Input: part model. Units: mm. Frame: model coordinates. A direction names the side the tool comes from. Coordinates: 2 decimals unless noted, no trailing zeros. Order: outer loops, then holes, each group sorted by start corner. A loop starts at its lowest first (then second) coordinate and runs counter-clockwise, first axis right, second up.
Autodesk Inventor part; units mm, degrees
ref_plane "YZ Plane" through (0, 0, 0) normal (1, 0, 0) x (0, 1, 0)
ref_plane "XZ Plane" through (0, 0, 0) normal (0, 1, 0) x (-1, 0, 0)
ref_plane "XY Plane" through (0, 0, 0) normal (0, 0, 1) x (1, 0, 0)
sketch "Sketch1" plane through (0, 0, 0) normal (0, 0, 1) x (1, 0, 0)
  circle A0 centre (0, 0) radius 50
  dimension "d0" = 100
extrude "Extrusion1" add sketch "Sketch1" along normal mid plane 100
sketch "Sketch2" plane through (0, 0, -50) normal (0, 0, -1) x (-1, 0, 0)
  circle A0 centre (0, 0) radius 45
  dimension "d3" = 90
extrude "Extrusion2" cut sketch "Sketch2" against normal blind 95
sketch "Sketch5" plane through (0, 0, 50) normal (0, 0, 1) x (1, 0, 0)
  point P0 (0, 0)
sketch "Sketch7" plane through (0, 0, 50) normal (0, 0, 1) x (1, 0, 0)
  arc A0 (50, 0) -> (50, 0) centre (0, 0) ccw construction
  circle A1 centre (0, 0) radius 50 construction
sketch "Sketch8" plane through (0, 0, -50) normal (0, 0, -1) x (-1, 0, 0)
  arc A0 (48.2963, -12.941) -> (48.2963, 12.941) centre (0, 0) ccw
  line L0 (0, 0) -> (50, 0) construction
  line L1 (48.2963, 12.941) -> (68.2963, 12.941)
  line L2 (68.2963, 12.941) -> (68.2963, -12.941)
  line L3 (68.2963, -12.941) -> (48.2963, -12.941)
  line L4 (48.2963, 12.941) -> (-48.2963, 12.941) construction
  line L5 (48.2963, -12.941) -> (-48.2963, -12.941) construction
  circle A1 centre (0, 0) radius 50 construction
  arc A2 (-48.2963, 12.941) -> (-48.2963, -12.941) centre (0, 0) ccw
  line L6 (-48.2963, -12.941) -> (-68.2963, -12.941)
  line L7 (-68.2963, -12.941) -> (-68.2963, 12.941)
  line L8 (-68.2963, 12.941) -> (-48.2963, 12.941)
  dimension "d31" = 50
  dimension "d34" = 20
  dimension "d35" = 20
extrude "Extrusion5" add sketch "Sketch8" against normal blind 10
sketch "Sketch9" plane through (0, 0, 50) normal (0, 0, 1) x (1, 0, 0)
  point P0 (0, 0)
sketch "Sketch10" plane through (0, 0, 50) normal (0, 0, 1) x (1, 0, 0)
  line L0 (-68.2963, -12.941) -> (-68.2963, 12.941) construction
  line L1 (-68.2963, -12.941) -> (-48.4721, 12.941) construction
  line L2 (-68.2963, 12.941) -> (-48.4721, -12.941) construction
  line L3 (48.2963, 12.941) -> (68.2963, 12.941) construction
  line L4 (48.2963, -12.941) -> (68.2963, 12.941) construction
  line L5 (68.2963, 12.941) -> (68.2963, -12.941) construction
  arc A0 (48.2963, -12.941) -> (48.2963, 12.941) centre (0, 0) ccw construction
  line L6 (68.2963, -12.941) -> (48.2963, 12.941) construction
  point P0 (-58.3842, 0)
  point P1 (58.2963, 0)
hole "Hole2" at (-58.3842, 0, 50) at (58.2963, 0, 50) direction (0, 0, -1) diameter 8 end through all counterbore diameter 11 counterbore depth 6.5
sketch "Sketch11" plane through (-68.2963, -12.941, -50) normal (0, -1, 0) x (1, 0, 0)
  line L0 (20, 0) -> (116.5926, 0) construction
  line L1 (118.2963, 100) -> (18.2963, 100) construction
  line L2 (20, 0) -> (118.2963, 100) construction
  line L3 (118.2963, 100) -> (18.2963, 100) construction
  line L4 (116.5926, 10) -> (116.5926, 0) construction
  line L5 (18.2963, 100) -> (116.5926, 0) construction
  point P0 (68.2963, 50)
  point P1 (68.2963, 50)
hole "Hole3" at (0, -12.941, 0) direction (0, 1, 0) diameter 8 end through all
sketch "Sketch12" plane through (0, 0, 50) normal (0, 0, 1) x (1, 0, 0)
  circle A0 centre (0, 0) radius 42
  circle A1 centre (0, 0) radius 25
  line L0 (0, 70.0025) -> (0, -70.0004)
  line L1 (-95.6148, 0) -> (95.6148, 0)
  point P0 (0, 25)
  point P1 (0, -25)
  dimension "d52" = 84
  dimension "d53" = 50
hole "Hole4" at (0, 25, 50) at (0, -25, 50) direction (0, 0, -1) diameter 6.4 end through all
sketch "Sketch13" plane through (0, 0, 50) normal (0, 0, 1) x (1, 0, 0)
  circle A0 centre (0, 0) radius 34
  line L0 (0, 70.0025) -> (0, -70.0004)
  line L1 (-95.6148, 0) -> (95.6148, 0)
  point P0 (-34, 0)
  point P1 (34, 0)
  dimension "d61" = 68
hole "Hole5" at (-34, 0, 50) at (34, 0, 50) direction (0, 0, -1) diameter 6.4 end through all
sketch "Sketch14" plane through (0, 0, 50) normal (0, 0, 1) x (1, 0, 0)
  circle A0 centre (0, 0) radius 25
  line L0 (0, 0) -> (-11.4805, -27.7164)
  line L1 (0, 70.0025) -> (0, -70.0004)
  line L2 (-95.6148, 0) -> (95.6148, 0)
  dimension "d69" = 50
  dimension "d70" = 30
hole "Hole6" at (-11.4805, -27.7164, 50) direction (0, 0, -1) diameter 6.4 end through all
sketch "Sketch15" plane through (0, 0, 50) normal (0, 0, 1) x (1, 0, 0)
  circle A0 centre (0, 0) radius 25 construction
  line L0 (0, 0) -> (-16.0697, 19.1511) construction
  line L1 (0, 70.0025) -> (0, -70.0004) construction
  line L2 (-95.6148, 0) -> (95.6148, 0) construction
  dimension "d79" = 50
  dimension "d80" = 40
hole "Hole7" at (-16.0697, 19.1511, 50) at (-16.0697, 19.1511, 50) direction (0, 0, -1) diameter 6.4 end through all
properties part number "Hus_Til_Motor"
Item 1: Cut plane C-C on x = -34. Return loops of the section in (y, z).
Response values:
outline: (-36.66, -50) - (-29.48, -50) - (-29.48, 45) - (-3.2, 45) - (-3.2, 50) - (-36.66, 50) - close; (3.2, 45) - (29.48, 45) - (29.48, -50) - (36.66, -50) - (36.66, 50) - (3.2, 50) - close
Item 2: Access query for faces 5 (the face through (3.905, 47.447, 0.867)), 6 (the face through (-58, -12.941, -45)), 7 (the face through (1, 1, 45)), 8 (the face through (-58, 12.941, -45)). Directions: +Z, -Z, +X, -X, +Y, -Y. A direction counts if a zero-diameter tool reaches every point of the face in a straight line with its end or side. Return the directions, or none.
Response values:
face 5: +Y
face 6: +Z, -Z, -X, -Y
face 7: -Z
face 8: +Z, -Z, -X, +Y
Item 3: Pin query (flat end, axial travel): pin 1 Ø2 at (x, z) = (34, -31.5) entering from -Y; pin 2 Ø4 at (x, y) = (-6.5, 13.5) entering from -Z; pin 3 Ø3 at (x, z) = (-59.5, -46.5) entering from +Y. Return the tip coordinate at first contact, or that it passes through.
Response values:
pin 1: stops at y = -37.56
pin 2: stops at z = 45
pin 3: stops at y = 12.94
Item 4: Cut plane A-A on y = 0. Return loops of the section in (x, z), then the cut area to 3 significant figures.
Response values:
outline: (-68.3, -50) - (-62.38, -50) - (-62.38, -40) - (-68.3, -40) - close; (-54.38, -50) - (-45, -50) - (-45, 45) - (-37.2, 45) - (-37.2, 50) - (-50, 50) - (-50, -40) - (-54.38, -40) - close; (-30.8, 45) - (30.8, 45) - (30.8, 50) - (-30.8, 50) - close; (37.2, 45) - (45, 45) - (45, -50) - (54.3, -50) - (54.3, -40) - (50, -40) - (50, 50) - (37.2, 50) - close; (62.3, -50) - (68.3, -50) - (68.3, -40) - (62.3, -40) - close
area: 1,590 mm2
Item 5: Ray query, probe 1 along Y at (x, z) = (0, 46.8); probe 2 along Z at (x, y) = (0, 46.7); probe 3 along Z at (x, y) = (30, 2.5). Return the intervals inside material, ascending.
Response values:
probe 1: y = -50 to -28.2, -21.8 to 21.8, 28.2 to 50
probe 2: z = -50 to -4, 4 to 50
probe 3: z = 45 to 50
Item 6: Draft query along Y for faces 1 (the face through (-37.173, 0.417, 47.465)), 2 (the face through (58, -12.941, -45)), 3 (the face through (-68.296, 0, -45)), 4 (the face through (47.69, -15.02, -0.7)). Return one class per face: pulls with the +Y half, pulls with the -Y half, needs draft (parallel to the pull), parting line crosses it, or undercut.
Response values:
face 1: undercut
face 2: pulls with the -Y half
face 3: needs draft
face 4: parting line crosses it
Item 7: Cut plane D-D on z = -26. Return loops of the section in (x, y), then the cut area to 3 significant figures.
Response values:
outline: circle Ø100 at (0, 0); hole circle Ø90 at (0, 0)
area: 1,490 mm2
Item 8: Cut plane B-B on y = 20. Return loops of the section in (x, z), then the cut area to 3 significant figures.
Response values:
outline: (-45.83, -50) - (-40.31, -50) - (-40.31, 45) - (-19.16, 45) - (-19.16, 50) - (-45.83, 50) - close; (-12.98, 45) - (40.31, 45) - (40.31, -50) - (45.83, -50) - (45.83, 50) - (-12.98, 50) - close
area: 1,480 mm2
